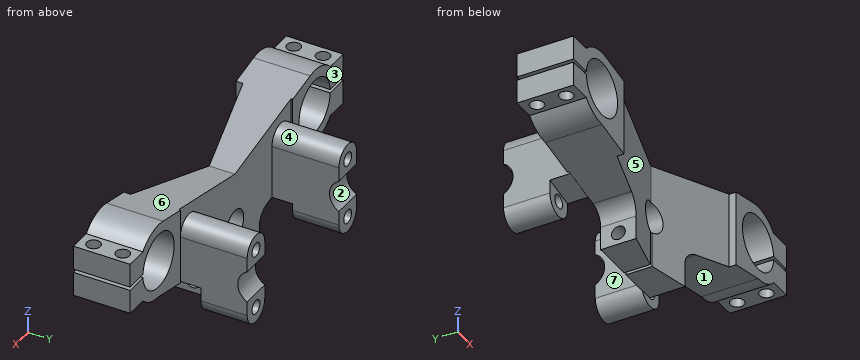
from build123d import *

# Parameters (mm, degrees)
BOSS_EXTRUDE1_DEPTH     = 33
FILLET2_R               = 10
FILLET3_R               = 10
CUT_EXTRUDE1_DEPTH      = 127.78010009
CUT_EXTRUDE1_DEPTH_BACK = 127.78010009
SKETCH3_W               = 115
SKETCH3_H               = 4.910725557
BOSS_EXTRUDE3_DEPTH     = 39
CUT_EXTRUDE5_DEPTH      = 65.5
CUT_EXTRUDE6_DEPTH      = 44
SKETCH9_R               = 4
CUT_EXTRUDE7_DEPTH      = 44
SKETCH10_R              = 4
CUT_EXTRUDE8_DEPTH      = 22
SKETCH11_R              = 4
CUT_EXTRUDE9_DEPTH      = 31
SKETCH12_R              = 10.5
CUT_EXTRUDE10_DEPTH     = 106.5


with BuildPart() as part:
    # Sketch1 → Boss-Extrude1 (new body)
    with BuildSketch(Plane(origin=(0, 0, 0), x_dir=(1, 0, 0), z_dir=(0, 1, 0))):
        with BuildLine():
            Line((-25, 55.5), (-25, 33.696074146))
            Line((-25, 33.696074146), (-80, 22.008574146))
            ThreePointArc((-80, 22.008574146), (-88.782047704, 20.180509757), (-96.105195929, 15))
            Line((-96.105195929, 15), (-109.105195929, 15))
            Line((-109.105195929, 15), (-109.105195929, 1))
            Line((-109.105195929, 1), (-95.968719423, 1))
            ThreePointArc((-95.968719423, 1), (-64, 0), (-95.968719423, -1))
            Line((-95.968719423, -1), (-109.105195929, -1))
            Line((-109.105195929, -1), (-109.105195929, -15))
            Line((-109.105195929, -15), (-96.105195929, -15))
            ThreePointArc((-96.105195929, -15), (-86.625068957, -20.987753506), (-75.425325161, -21.527881597))
            Line((-75.425325161, -21.527881597), (0, -5.5))
            Line((0, -5.5), (75.425325161, -21.527881597))
            ThreePointArc((75.425325161, -21.527881597), (86.625068957, -20.987753506), (96.105195929, -15))
            Line((96.105195929, -15), (109.105195929, -15))
            Line((109.105195929, -15), (109.105195929, -1))
            Line((109.105195929, -1), (95.968719423, -1))
            ThreePointArc((95.968719423, -1), (64, 0), (95.968719423, 1))
            Line((95.968719423, 1), (109.105195929, 1))
            Line((109.105195929, 1), (109.105195929, 15))
            Line((109.105195929, 15), (96.105195929, 15))
            ThreePointArc((96.105195929, 15), (88.782047704, 20.180509757), (80, 22.008574146))
            Line((80, 22.008574146), (25, 33.696074146))
            Line((25, 33.696074146), (25, 55.5))
            Line((25, 55.5), (1, 55.5))
            Line((1, 55.5), (1, 34.94427191))
            ThreePointArc((1, 34.94427191), (0, 17), (-1, 34.94427191))
            Line((-1, 34.94427191), (-1, 55.5))
            Line((-1, 55.5), (-25, 55.5))
        make_face()
    extrude(amount=BOSS_EXTRUDE1_DEPTH)

    # Fillet2
    fillet2_edges = [part.edges().sort_by_distance(p)[0] for p in [
        (25, 16.5, -33.696074146),
    ]]
    fillet(fillet2_edges, radius=FILLET2_R)

    # Fillet3
    fillet3_edges = [part.edges().sort_by_distance(p)[0] for p in [
        (-25, 16.5, -33.696074146),
    ]]
    fillet(fillet3_edges, radius=FILLET3_R)

    # Sketch3 → Cut-Extrude1 (cut, two sides: drawn at the far end of the back side and taken through both)
    with BuildSketch(Plane.XY.offset(-CUT_EXTRUDE1_DEPTH_BACK)):
        with Locations((0, 34.455362779)):
            Rectangle(SKETCH3_W, SKETCH3_H)
        Polygon((-57.5, 4), (-57.5, -3.298292375), (57.5, -3.298292375), (57.5, 4), (0, 17), align=None)
    extrude(amount=CUT_EXTRUDE1_DEPTH + CUT_EXTRUDE1_DEPTH_BACK, mode=Mode.SUBTRACT)

    # Sketch5 → Boss-Extrude3 (add)
    with BuildSketch(Plane(origin=(0, 71, 0), x_dir=(1, 0, 0), z_dir=(0, 1, 0))):
        with BuildLine():
            Line((-38, 0), (-38, 35))
            ThreePointArc((-38, 35), (-47, 44), (-56, 35))
            Line((-56, 35), (-56, 0))
            ThreePointArc((-56, 0), (-47, -9), (-38, 0))
        make_face()
        with BuildLine():
            Line((56, 0), (56, 35))
            ThreePointArc((56, 35), (47, 44), (38, 35))
            Line((38, 35), (38, 0))
            ThreePointArc((38, 0), (47, -9), (56, 0))
        make_face()
    extrude(amount=-BOSS_EXTRUDE3_DEPTH)

    # Sketch6 → Cut-Extrude5 (cut, symmetric)
    with BuildSketch(Plane(origin=(0, 0, 0), x_dir=(0, 0, -1), z_dir=(1, 0, 0))):
        Polygon((44, 71), (44, 44), (31.054287073, 44), (31.054287073, 32), (44, 32), (62.918124126, 32), (62.918124126, 71), align=None)
    extrude(amount=CUT_EXTRUDE5_DEPTH, both=True, mode=Mode.SUBTRACT)

    # Sketch7 → Cut-Extrude6 (cut)
    with BuildSketch(Plane(origin=(0, 0, 0), x_dir=(1, 0, 0), z_dir=(0, 1, 0))):
        Polygon((-56, 31.054287073), (-38, 31.054287073), (-56, 27.108574146), align=None)
        Polygon((56, 27.108574146), (56, 31.054287073), (38, 31.054287073), align=None)
    extrude(amount=CUT_EXTRUDE6_DEPTH, mode=Mode.SUBTRACT)

    # Sketch9 → Cut-Extrude7 (cut)
    with BuildSketch(Plane(origin=(0, 71, 0), x_dir=(1, 0, 0), z_dir=(0, 1, 0))):
        with Locations(Location((-47, 0, 0), (0, 0, 270))):
            Circle(SKETCH9_R)
        with Locations(Location((-47, 35, 0), (0, 0, 270))):
            Circle(SKETCH9_R)
        with Locations(Location((47, 0, 0), (0, 0, 270))):
            Circle(SKETCH9_R)
        with Locations(Location((47, 35, 0), (0, 0, 270))):
            Circle(SKETCH9_R)
    extrude(amount=-CUT_EXTRUDE7_DEPTH, mode=Mode.SUBTRACT)

    # Sketch10 → Cut-Extrude8 (cut, symmetric)
    with BuildSketch(Plane.XY):
        with Locations((-102.605195929, 8)):
            Circle(SKETCH10_R)
        with Locations((-102.605195929, 25)):
            Circle(SKETCH10_R)
        with Locations((102.605195929, 8)):
            Circle(SKETCH10_R)
        with Locations((102.605195929, 25)):
            Circle(SKETCH10_R)
    extrude(amount=CUT_EXTRUDE8_DEPTH, both=True, mode=Mode.SUBTRACT)

    # Sketch11 → Cut-Extrude9 (cut, symmetric)
    with BuildSketch(Plane(origin=(0, 0, 0), x_dir=(0, 0, -1), z_dir=(1, 0, 0))):
        with Locations((48.647181255, 21.673913043)):
            Circle(SKETCH11_R)
    extrude(amount=CUT_EXTRUDE9_DEPTH, both=True, mode=Mode.SUBTRACT)

    # Sketch12 → Cut-Extrude10 (cut, symmetric)
    with BuildSketch(Plane(origin=(0, 0, 0), x_dir=(0, 0, -1), z_dir=(1, 0, 0))):
        with Locations((17.5, 76)):
            Circle(SKETCH12_R)
    extrude(amount=CUT_EXTRUDE10_DEPTH, both=True, mode=Mode.SUBTRACT)


solid = part.part
Can you work these out from the model? Positions are in its coordinate system, mm. Face numbers are marked on the shaded views. A direction names the side the tool comes from. Coordinates: 2 decimals unless noted, no trailing zeros. Write each loop counter-clockwise with the first axis right and the second up, starting at its lowest first coordinate (ties: lowest second). Pieces come first, ordered by that corner, then holes. Notation, with made-up numbers: (3, 1.5) -> (44, 1.5) arc R13 ccw to (44, 8.5) -> close; hole circle Ø10 at (-2.5, -11.5). An arc over 180 degrees is marked (long way). Write each question's results on one line, items separated by ' | '. Start each with the question number.
Item 1: On a 3-axis mill with a long thin cutter (end or side, diameter ignored), from which of +Z, -Z, +X, -X, +Y, -Y can I reach the whole of each face in a straight line? I mean the marked faces 4, 5, 6 and 7. Say none if no direction works.
Item 2: Please list where these lines run through material, in increasing order: probe 1 along X at (y, z) = (51.75, -35); probe 2 along X at (y, z) = (57, -30.5); probe 3 along Z at (x, y) = (3, 20.5).
Item 3: If we section it at B-B, the plane z = 11: Write out the boundary of the cut face in (x, y), and give its area (3 significant figures).
Item 4: I'm going to push flat-ended pins straight in: P1, Ø12, axis at y = 28, z = -42.5, coming from the -X side; P2, Ø4, axis at x = -37, y = 53, coming from the +Z side; P3, Ø9, axis at x = 47, z = -35, coming from the -Y side. Where does each tip first touch, or does it pass through?
Item 5: If we section it at D-D, the plane x = -78: Write out the boundary of the cut face in (y, z), and give its area (3 significant figures).
Item 6: If we section it at A-A, the plane y = 38: Write out the boundary of the cut face in (x, z), and give its area (3 significant figures).
Item 7: Thinking about a two-plate mould opening in Z: for the marked faces 1, 2 and 3, which applies, released by +Z, released by -Z, zero draft, split by the parting line, or undercut?
Item 8: If we section it at C-C, the plane x = -6: Write out the boundary of the cut face in (y, z) (3 decimals), and give its area (3 significant figures).
Answer block:
1) face 4: +Z, +Y | face 5: +Z, -Z, -Y | face 6: +Z, +Y, -Y | face 7: +Z, -Z, +Y
2) probe 1: -56 to -51, -43 to -38, 38 to 43, 51 to 56 | probe 2: -56 to -38, 38 to 56 | probe 3: -55.5 to -52.47, -44.82 to -34.49, -17.51 to 6.14
3) outline: (-109.11, 0) -> (-91.62, 0) -> (-91.62, 33) -> (-109.11, 33) -> close; (-68.38, 0) -> (-57.5, 0) -> (-57.5, 4) -> (-25.88, 11.15) -> (-25.88, 32) -> (-57.5, 32) -> (-57.5, 33) -> (-68.38, 33) -> close; (25.88, 11.15) -> (57.5, 4) -> (57.5, 0) -> (68.38, 0) -> (68.38, 33) -> (57.5, 33) -> (57.5, 32) -> (25.88, 32) -> close; (91.62, 0) -> (109.11, 0) -> (109.11, 33) -> (91.62, 33) -> close; hole circle Ø8 at (-102.61, 8); hole circle Ø8 at (-102.61, 25); hole circle Ø8 at (102.61, 8); hole circle Ø8 at (102.61, 25) | area: 3,220 mm²
4) P1: x = -26.52 | P2: z = 4.12 | P3: y = 44
5) outline: (0, -22.43) -> (33, -22.43) -> (33, -15.87) -> (0, -15.87) -> close; (0, 15.87) -> (33, 15.87) -> (33, 21.92) -> (0, 21.92) -> close | area: 416 mm²
6) outline: (-56, -27.11) -> (-38, -31.05) -> (-38, 0) arc R9 ccw to (-56, 0) -> close; (38, -31.05) -> (56, -27.11) -> (56, 0) arc R9 ccw to (38, 0) -> close; hole circle Ø8 at (-47, 0); hole circle Ø8 at (47, 0) | area: 1,200 mm²
7) face 1: released by -Z | face 2: undercut | face 3: zero draft
8) outline: (15.643, -55.5) -> (32, -55.5) -> (32, -32.708) -> (15.643, -32.708) -> close; (15.643, -19.292) -> (32, -19.292) -> (32, 6.775) -> (15.643, 6.775) -> close; hole circle Ø8 at (21.674, -48.647) | area: 749 mm²
